```python
from build123d import *

# Parameters (mm, degrees)
SKETCH1_W           = 50
SKETCH1_H           = 39
SKETCH1_R           = 2.75
SKETCH1_R_2         = 2.3
BOSS_EXTRUDE1_DEPTH = 7
CUT_EXTRUDE1_DEPTH  = 4.2
FILLET1_R           = 5
SKETCH3_W           = 8
SKETCH3_H           = 5
BOSS_EXTRUDE2_DEPTH = 4
FILLET2_R           = 1
FILLET3_R           = 1
FILLET4_R           = 1


with BuildPart() as part:
    # Sketch1 → Boss-Extrude1 (new body)
    with BuildSketch(Plane.XY):
        Rectangle(SKETCH1_W, SKETCH1_H)
        with Locations((-17, 0)):
            Circle(SKETCH1_R, mode=Mode.SUBTRACT)
        with Locations((20, 10)):
            Circle(SKETCH1_R_2, mode=Mode.SUBTRACT)
        with Locations((20, -10)):
            Circle(SKETCH1_R_2, mode=Mode.SUBTRACT)
    extrude(amount=BOSS_EXTRUDE1_DEPTH)

    # Sketch2 → Cut-Extrude1 (cut)
    with BuildSketch(Plane(origin=(0, 0, 0), x_dir=(-1, 0, 0), z_dir=(0, 0, -1))):
        Polygon((17, 4.67653718), (12.95, 2.33826859), (12.95, -2.33826859), (17, -4.67653718), (21.05, -2.33826859), (21.05, 2.33826859), align=None)
    extrude(amount=-CUT_EXTRUDE1_DEPTH, mode=Mode.SUBTRACT)

    # Fillet1
    fillet1_edges = [part.edges().sort_by_distance(p)[0] for p in [
        (25, -19.5, 3.5),
        (-25, -19.5, 3.5),
        (-25, 19.5, 3.5),
        (25, 19.5, 3.5),
    ]]
    fillet(fillet1_edges, radius=FILLET1_R)

    # Sketch3 → Boss-Extrude2 (add)
    with BuildSketch(Plane(origin=(0, 0, 0), x_dir=(-1, 0, 0), z_dir=(0, 0, -1))):
        with Locations((-12.5, 10)):
            Rectangle(SKETCH3_W, SKETCH3_H)
    boss_extrude2 = extrude(amount=BOSS_EXTRUDE2_DEPTH)

    # Mirror1: Boss-Extrude2 across plane
    add(boss_extrude2.mirror(Plane.ZX))

    # Fillet2
    fillet2_edges = [part.edges().sort_by_distance(p)[0] for p in [
        (8.5, 7.5, -2),
        (8.5, 12.5, -2),
        (16.5, 12.5, -2),
        (16.5, 7.5, -2),
    ]]
    fillet(fillet2_edges, radius=FILLET2_R)

    # Fillet3
    fillet3_edges = [part.edges().sort_by_distance(p)[0] for p in [
        (8.5, -12.5, -2),
        (8.5, -7.5, -2),
        (16.5, -7.5, -2),
        (16.5, -12.5, -2),
    ]]
    fillet(fillet3_edges, radius=FILLET3_R)

    # Fillet4
    fillet4_edges = [part.edges().sort_by_distance(p)[0] for p in [
        (25, 0, 7),
        (0, -19.5, 7),
        (0, 19.5, 7),
        (-25, 0, 7),
        (23.535533906, 18.035533906, 7),
        (-23.535533906, 18.035533906, 7),
        (-23.535533906, -18.035533906, 7),
        (23.535533906, -18.035533906, 7),
    ]]
    fillet(fillet4_edges, radius=FILLET4_R)


solid = part.part
```
Design review of the part built by this model. Coordinates are the model's own, in mm. A direction names the side the tool comes from. Coordinates: 2 decimals unless noted, no trailing zeros. Order: outer loops, then holes, each group sorted by start corner. A loop starts at its lowest first (then second) coordinate and runs counter-clockwise, first axis right, second up.
1) Clearance check with flat-ended pins moving along their axes: pin 1 (4.5 mm diameter, centred on x = -17, y = 0, fed in from +Z); pin 2 (3 mm diameter, centred on x = -16.5, y = 2.5, fed in from -Z); pin 3 (1.5 mm diameter, centred on y = -9.5, z = -2.5, fed in from +X); pin 4 (11.5 mm diameter, centred on x = -1.5, y = 5.5, fed in from -Z). State where each tip first meets the part, or that it passes through.
2) Take a section at C-C, the plane z = -1. Give the boundary of the cut face in (x, y).
3) For faces 1 (the flat face through (13, 12.5, -2)), 2 (the cylindrical face through (8.801, 12.215, -2.028)), 3 (the cylindrical face through (16.199, -7.785, -2.028)), 4 (the flat face through (8.5, 10, -2)), list the 3-axis set-ups (+Z, -Z, +X, -X, +Y, -Y) from which the entire face can be reached by the end or side of a thin tool; tool diameter is ignored.
4) Wall thickness on line 1 along Y through (x, z) = (20, 3.75); line 2 along X through (y, z) = (0, 6); line 3 along Y through (x, z) = (-17, 5.2): over which ranges is each line inside the solid? List them lowest first.
5) Take a section at A-A, the plane z = 1.75. Give the boundary of the cut face in (x, y).
6) Take a section at D-D, the plane x = 14.5. Give the boundary of the cut face in (y, z), and give its area (3 significant figures).
7) Take a section at B-B, the plane y = 10. Give the boundary of the cut face in (x, z), and give its area (3 significant figures).
8) Mouldability with a two-part tool opening along Y and no side actions: class faces 5 (the flat face through (-15, 3.52, 2.07)), 6 (the cylindrical face through (-0.28, 19.215, 6.699)), 7 (the flat face through (-19, -3.52, 2.07)), 8 (the flat face through (16.5, -10, -2)) as +Y half, -Y half, draft (parallel to the pull), parting line (faces both ways), or undercut.
Returned:
1. pin 1: passes through
1. pin 2: stops at z = 4.2
1. pin 3: stops at x = 16.5
1. pin 4: stops at z = 0
2. outline: (8.5, -11.5) arc R1 ccw to (9.5, -12.5) - (15.5, -12.5) arc R1 ccw to (16.5, -11.5) - (16.5, -8.5) arc R1 ccw to (15.5, -7.5) - (9.5, -7.5) arc R1 ccw to (8.5, -8.5) - close; (8.5, 8.5) arc R1 ccw to (9.5, 7.5) - (15.5, 7.5) arc R1 ccw to (16.5, 8.5) - (16.5, 11.5) arc R1 ccw to (15.5, 12.5) - (9.5, 12.5) arc R1 ccw to (8.5, 11.5) - close
3. face 1: -Z, +X, -X, +Y
3. face 2: -Z, -X, +Y
3. face 3: -Z, +X
3. face 4: -Z, -X, +Y, -Y
4. line 1: y = -19.5 to -12.3, -7.7 to 7.7, 12.3 to 19.5
4. line 2: x = -25 to -19.75, -14.25 to 25
4. line 3: y = -19.5 to -2.75, 2.75 to 19.5
5. outline: (-25, -14.5) arc R5 ccw to (-20, -19.5) - (20, -19.5) arc R5 ccw to (25, -14.5) - (25, 14.5) arc R5 ccw to (20, 19.5) - (-20, 19.5) arc R5 ccw to (-25, 14.5) - close; hole (-21.05, -2.34) - (-17, -4.68) - (-12.95, -2.34) - (-12.95, 2.34) - (-17, 4.68) - (-21.05, 2.34) - close; hole circle Ø4.6 at (20, -10); hole circle Ø4.6 at (20, 10)
6. outline: (-19.5, 0) - (-12.5, 0) - (-12.5, -4) - (-7.5, -4) - (-7.5, 0) - (7.5, 0) - (7.5, -4) - (12.5, -4) - (12.5, 0) - (19.5, 0) - (19.5, 6) arc R1 ccw to (18.5, 7) - (-18.5, 7) arc R1 ccw to (-19.5, 6) - close
6. area: 313 mm2
7. outline: (-25, 0) - (8.5, 0) - (8.5, -4) - (16.5, -4) - (16.5, 0) - (17.7, 0) - (17.7, 7) - (-24, 7) arc R1 ccw to (-25, 6) - close; (22.3, 0) - (25, 0) - (25, 6) arc R1 ccw to (24, 7) - (22.3, 7) - close
7. area: 349 mm2
8. face 5: undercut
8. face 6: +Y half
8. face 7: undercut
8. face 8: draft
